from build123d import *

# Parameters (mm, degrees)
SKETCH1_W           = 171.45
SKETCH1_H           = 171.45
BOSS_EXTRUDE1_DEPTH = 18.25625
SKETCH2_R           = 17.4625
CUT_EXTRUDE1_DEPTH  = 123.60033407
SKETCH5_R           = 38.1
CUT_EXTRUDE2_DEPTH  = 123.60033407


with BuildPart() as part:
    # Sketch1 → Boss-Extrude1 (new body)
    with BuildSketch(Plane(origin=(0, 0, 0), x_dir=(1, 0, 0), z_dir=(0, 1, 0))):
        Rectangle(SKETCH1_W, SKETCH1_H)
    extrude(amount=BOSS_EXTRUDE1_DEPTH)

    # Sketch2 → Cut-Extrude1 (cut, through all)
    with BuildSketch(Plane(origin=(0, 18.25625, 0), x_dir=(1, 0, 0), z_dir=(0, 1, 0))):
        with Locations((-76.2, 76.2)):
            Circle(SKETCH2_R)
        with Locations((76.2, 76.2)):
            Circle(SKETCH2_R)
        with Locations((76.2, -76.2)):
            Circle(SKETCH2_R)
        with Locations((-76.2, -76.2)):
            Circle(SKETCH2_R)
    extrude(amount=-CUT_EXTRUDE1_DEPTH, mode=Mode.SUBTRACT)

    # Sketch5 → Cut-Extrude2 (cut, through all)
    with BuildSketch(Plane(origin=(0, 18.25625, 0), x_dir=(1, 0, 0), z_dir=(0, 1, 0))):
        with Locations(Location((0, 0, 0), (0, 0, 270))):
            Circle(SKETCH5_R)
    extrude(amount=-CUT_EXTRUDE2_DEPTH, mode=Mode.SUBTRACT)


solid = part.part
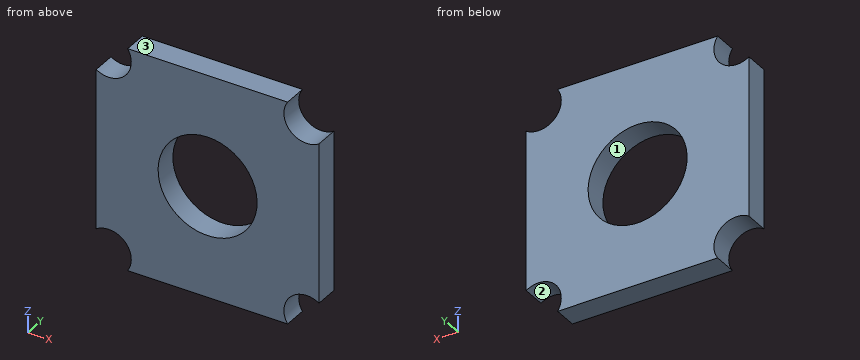
Can you work these out from the model? Positions are in its coordinate system, mm. Face numbers are marked on the shaded views. Give positions to 0.01 mm unless a question says otherwise; leave off trailing zeros. Loops run counter-clockwise (first coordinate to the right, second up) from the corner with the lowest first, then second, coordinate; pieces in that order, holes last. Notation, with made-up numbers: M -6,23 L 30,23 A13 cw 30,38 Z; hole C 49.25,86.25 d8. An arc over 180 degrees is marked long. One line per item, written item: value.
1) Please list where these lines run through material, in increasing order: line 1 (X direction, y = 4.25, z = 0) (3 decimals); line 2 (Z direction, x = -10, y = 10.5) (3 decimals); line 3 (X direction, y = 17.75, z = -16) (3 decimals).
Geometry check:
line 1: x = -85.725 to -38.1, 38.1 to 85.725
line 2: z = -85.725 to -36.764, 36.764 to 85.725
line 3: x = -85.725 to -34.578, 34.578 to 85.725
2) Imagine slicing it at A-A on z = 0. Write out the boundary of the cut face in (x, y) (3 decimals), and give its area (3 significant figures).
Geometry check:
outline: M -85.725,0 L -38.1,0 L -38.1,18.256 L -85.725,18.256 Z; M 38.1,0 L 85.725,0 L 85.725,18.256 L 38.1,18.256 Z
area: 1,740 mm²
3) Imagine slicing it at C-C on y = 3.5. Write out the boundary of the cut face in (x, z) (1 decimal), and give its area (3 significant figures).
Geometry check:
outline: M -85.7,-61.6 A17.5 cw -61.6,-85.7 L 61.6,-85.7 A17.5 cw 85.7,-61.6 L 85.7,61.6 A17.5 cw 61.6,85.7 L -61.6,85.7 A17.5 cw -85.7,61.6 Z; hole C 0,0 d76.2
area: 22,300 mm²
4) Imagine slicing it at B-B on x = 0. Write out the boundary of the cut face in (y, z) (3 decimals).
Geometry check:
outline: M 0,-85.725 L 18.256,-85.725 L 18.256,-38.1 L 0,-38.1 Z; M 0,38.1 L 18.256,38.1 L 18.256,85.725 L 0,85.725 Z
5) Imagine slicing it at D-D on x = 64. Write out the boundary of the cut face in (y, z).
Geometry check:
outline: M 0,-63.71 L 18.26,-63.71 L 18.26,63.71 L 0,63.71 Z
6) Thinking about a two-plate mould opening in X: for the marked faces 1, 2 and 3, which applies, +X half, -X half, draft (parallel to the pull), parting line (faces both ways), or undercut?
Geometry check:
face 1: undercut
face 2: undercut
face 3: draft
